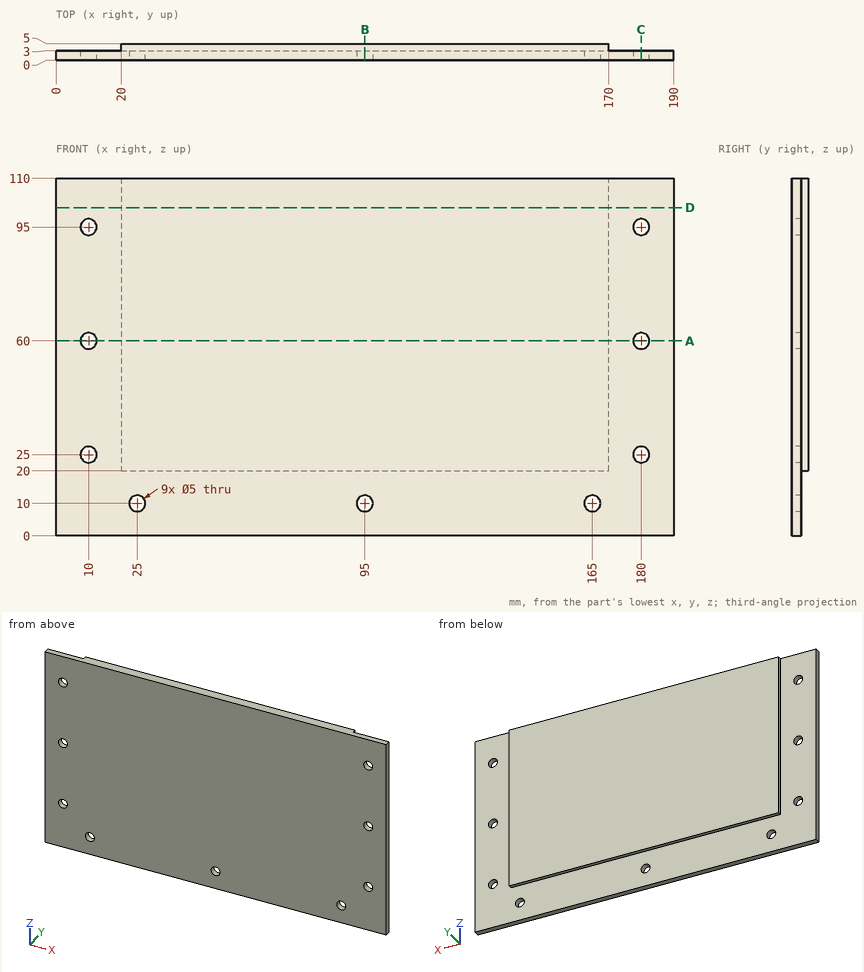
Job drawing, mm, ordinate dimensions from the low corner. One solid piece. Round coordinates to 2 decimals unless told otherwise and drop trailing zeros. Order: outer loops, then holes, each group sorted by start corner. A loop starts at its lowest first (then second) coordinate and runs counter-clockwise, first axis right, second up. Notation, with made-up numbers: M 20,86 L 48,86 A27 ccw 48,112 Z; hole C -39,-22 d8. An arc over 180 degrees is marked long. Write each question's results on one line, items separated by ' | '. Start each with the question number.
(1) Probe probe 1 along Z at (x, y) = (10, 1.45); probe 2 along Z at (x, y) = (25, 0.9); probe 3 along X at (y, z) = (3.05, 64). List the from-to ranges inside material, lowest first. Write a range as from..to.
(2) Drop flat-ended pins along their axis: pin 1 (6 mm diameter, centred on x = 180, z = 25, fed in from +Y); pin 2 (6 mm diameter, centred on x = 10, z = 60, fed in from -Y); pin 3 (1 mm diameter, centred on y = 4, z = 79, fed in from +X); pin 4 (4.5 mm diameter, centred on x = 180, z = 60, fed in from -Y). Give the stop position or say it passes through.
(3) Saw through at B-B, the plane x = 95. Give the cut face in (y, z).
(4) Saw through at C-C, the plane x = 180. Give the cut face in (y, z).
(5) Saw through at D-D, the plane z = 101. Give the cut face in (x, y), then the cut area to 3 significant figures.
(6) Saw through at A-A, the plane z = 60. Give the cut face in (x, y), then the cut area to 3 significant figures.
Established:
1) probe 1: z = 0..22.5, 27.5..57.5, 62.5..92.5, 97.5..110 | probe 2: z = 0..7.5, 12.5..110 | probe 3: x = 20..170
2) pin 1: stops at y = 3 | pin 2: stops at y = 0 | pin 3: stops at x = 170 | pin 4: passes through
3) outline: M 0,0 L 3,0 L 3,7.5 L 0,7.5 Z; M 0,12.5 L 3,12.5 L 3,20 L 5,20 L 5,110 L 0,110 Z
4) outline: M 0,0 L 3,0 L 3,22.5 L 0,22.5 Z; M 0,27.5 L 3,27.5 L 3,57.5 L 0,57.5 Z; M 0,62.5 L 3,62.5 L 3,92.5 L 0,92.5 Z; M 0,97.5 L 3,97.5 L 3,110 L 0,110 Z
5) outline: M 0,0 L 190,0 L 190,3 L 170,3 L 170,5 L 20,5 L 20,3 L 0,3 Z | area: 870 mm^2
6) outline: M 0,0 L 7.5,0 L 7.5,3 L 0,3 Z; M 12.5,0 L 177.5,0 L 177.5,3 L 170,3 L 170,5 L 20,5 L 20,3 L 12.5,3 Z; M 182.5,0 L 190,0 L 190,3 L 182.5,3 Z | area: 840 mm^2
